The figure shows three views and two pictorial views of one solid part (mm, origin at its lowest corner). Answer the questions. A direction names the side the tool comes from. Coordinates: 2 decimals unless noted, no trailing zeros. Loops run counter-clockwise (first coordinate to the right, second up) from the corner with the lowest first, then second, coordinate; pieces in that order, holes last.
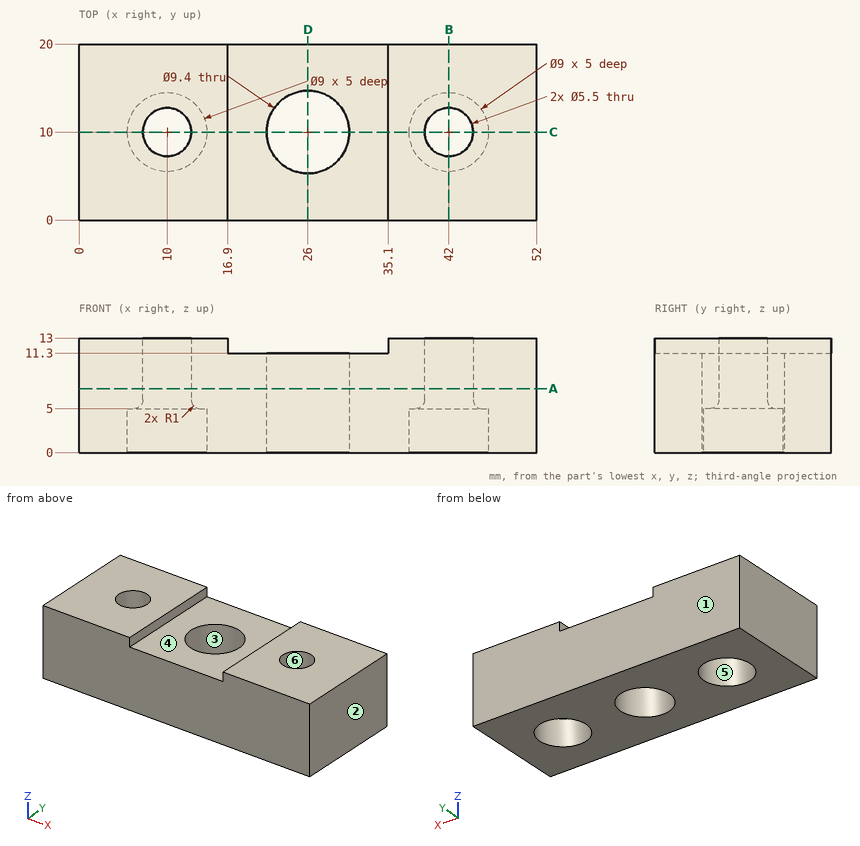
Q1. A cutting plane is placed at C-C (y = 10). Count the separate pieces of the cut face and the enclosed holes in it, then the cut area to 3 significant figures.
Findings below:
separate pieces: 4
enclosed holes: 0
area: 360 mm2
Q2. Straight lines are drawn through the part: probe 1 along X at (y, z) = (10, 11.5); probe 2 along Y at (x, z) = (42, 2.2); probe 3 along Y at (x, z) = (10, 9.5). For each, find the intervals that lie inside material, in ascending order.
Findings below:
probe 1: x = 0 to 7.25, 12.75 to 16.9, 35.1 to 39.25, 44.75 to 52
probe 2: y = 0 to 5.5, 14.5 to 20
probe 3: y = 0 to 7.25, 12.75 to 20
Q3. Which of the six approach directions +Z, -Z, +X, -X, +Y, -Y give full straight-line access (tool end or side, diameter ignored) to the marked faces 4, 5 and 6?
Findings below:
face 4: +Z, +Y, -Y
face 5: -Z
face 6: +Z, -Z
Q4. A cutting plane is placed at B-B (x = 42). Give the vertices of the cut face in (y, z).
Findings below:
outline: (0, 0) - (5.5, 0) - (5.5, 5) - (6.25, 5) arc R1 ccw to (7.25, 6) - (7.25, 13) - (0, 13) - close; (12.75, 6) arc R1 ccw to (13.75, 5) - (14.5, 5) - (14.5, 0) - (20, 0) - (20, 13) - (12.75, 13) - close
Q5. A cutting plane is placed at D-D (x = 26). Give the vertices of the cut face in (y, z), then the cut area to 3 significant figures.
Findings below:
outline: (0, 0) - (5.3, 0) - (5.3, 11.3) - (0, 11.3) - close; (14.7, 0) - (20, 0) - (20, 11.3) - (14.7, 11.3) - close
area: 120 mm2
Q6. Flat-ended cylindrical pins translate along their axes: pin 1 Ø12 at (x, y) = (26, 10) entering from +Z; pin 2 Ø2 at (x, y) = (32, 4) entering from -Z; pin 3 Ø6.5 at (x, y) = (42, 10) entering from -Z; pin 4 Ø4 at (x, y) = (26.5, 12) entering from -Z (3 decimals). Find the tip coordinate at first contact, or state that the pin passes through.
Findings below:
pin 1: stops at z = 11.3
pin 2: stops at z = 0
pin 3: stops at z = 5.13
pin 4: passes through
Q7. A cutting plane is placed at A-A (z = 7.25). Give the vertices of the cut face in (x, y).
Findings below:
outline: (0, 0) - (52, 0) - (52, 20) - (0, 20) - close; hole circle Ø5.5 at (10, 10); hole circle Ø9.4 at (26, 10); hole circle Ø5.5 at (42, 10)
Q8. Determine the mould class of the marked faces 1, 2 and 3 for opening direction X: +X half, -X half, draft (parallel to the pull), parting line (faces both ways), or undercut.
Findings below:
face 1: draft
face 2: +X half
face 3: undercut
